Part print with two shaded views. Sizes in mm from the minimum x, y, z corner. Give positions to 0.01 mm unless a question says otherwise; leave off trailing zeros. Loops run counter-clockwise (first coordinate to the right, second up) from the corner with the lowest first, then second, coordinate; pieces in that order, holes last. Notation, with made-up numbers: (80.25, -33) -> (131.25, -33) arc R7 cw to (131.25, -27) -> close; hole circle Ø5 at (5, 43). An arc over 180 degrees is marked (long way). One line per question, with ' | ' between items. Start each with the question number.
(1) Slice it at A-A, the plane y = 9. Write the cut outline in (x, z).
(2) Slice it at B-B, the plane z = 0.95. Write the cut outline in (x, y).
(3) Drill centre lines: L1, parallel to Y at x = 22.5, z = 0.4; L2, parallel to X at y = 22, z = 1.9; L3, parallel to X at y = 17, z = 2.05. Where is each one in solid material? Low to high. Write a range as from..to.
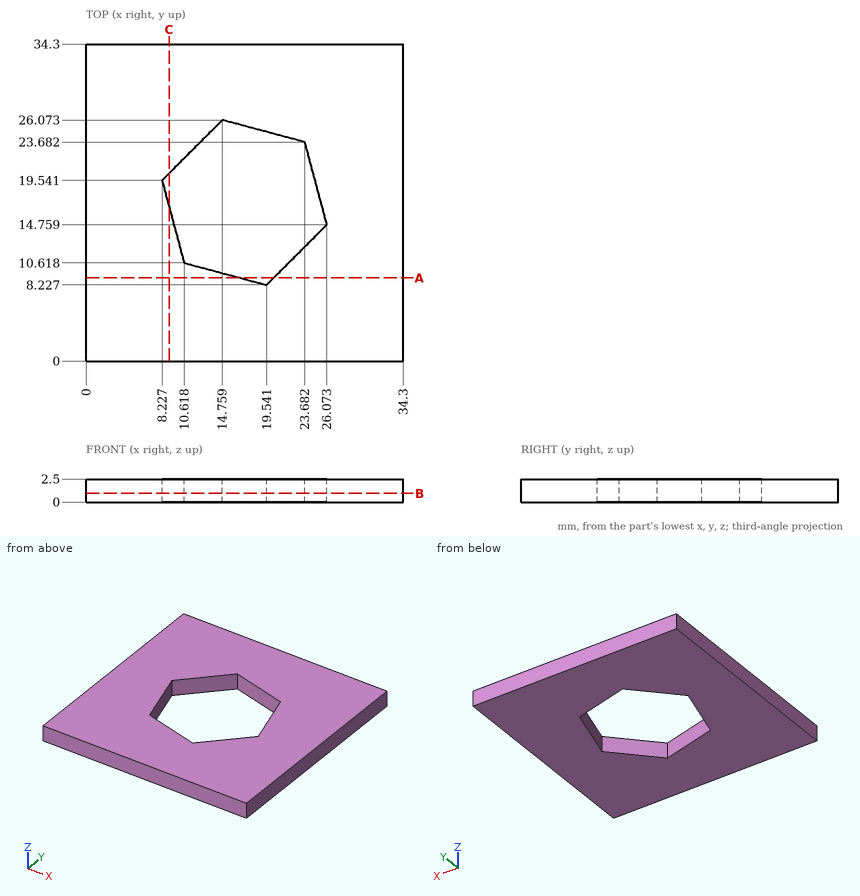
Final values:
1) outline: (0, 0) -> (16.66, 0) -> (16.66, 2.5) -> (0, 2.5) -> close; (20.31, 0) -> (34.3, 0) -> (34.3, 2.5) -> (20.31, 2.5) -> close
2) outline: (0, 0) -> (34.3, 0) -> (34.3, 34.3) -> (0, 34.3) -> close; hole (8.23, 19.54) -> (10.62, 10.62) -> (19.54, 8.23) -> (26.07, 14.76) -> (23.68, 23.68) -> (14.76, 26.07) -> close
3) L1: 0..11.19, 24..34.3 | L2: 0..10.69, 24.13..34.3 | L3: 0..8.91, 25.47..34.3
